```python
from build123d import *

# Parameters (mm, degrees)
F0_W        = 119.0486699343
F0_H        = 122.4547103047
F1_DEPTH    = 25.4
F2_T1_DEPTH = 131.7486699343
F2_T3_DEPTH = 135.1547103047
F3_T        = -5.08


# Not quite as in the source:
# - a fillet or chamfer that OpenCascade refuses, or shapes differently, is made with other operations: its cross-section is extruded or revolved along the edge and cut away or added


with BuildPart() as f1:
    # F0 (on Front) → F1 (new body)
    with BuildSketch(Plane.XZ):
        Rectangle(F0_W, F0_H)
    extrude(amount=F1_DEPTH)

    # F2: fillet of radius 2.54 on 4 edges, made by hand

    # F2_s2 → F2_t1 (cut)
    with BuildSketch(Plane.YZ.offset(-65.8743349671)):
        with BuildLine():
            add(Edge.make_bspline(
                [(-22.86, 61.2273551524), (-25.4, 61.2273551524), (-25.4, 58.6873551524)],
                knots=[0, 0, 0, 1, 1, 1], degree=2, weights=[1, 1, 1]))
            Line((-25.4, 58.6873551524), (-25.4, 61.2273551524))
            Line((-25.4, 61.2273551524), (-22.86, 61.2273551524))
        make_face()
        with BuildLine():
            add(Edge.make_bspline(
                [(-22.86, -61.2273551524), (-25.4, -61.2273551524), (-25.4, -58.6873551524)],
                knots=[0, 0, 0, 1, 1, 1], degree=2, weights=[1, 1, 1]))
            Line((-25.4, -58.6873551524), (-25.4, -61.2273551524))
            Line((-25.4, -61.2273551524), (-22.86, -61.2273551524))
        make_face()
    extrude(amount=F2_T1_DEPTH, mode=Mode.SUBTRACT)

    # F2_s4 → F2_t3 (cut)
    with BuildSketch(Plane.XY.offset(-67.5773551524)):
        with BuildLine():
            add(Edge.make_bspline(
                [(-59.5243349671, -22.86), (-59.5243349671, -25.4), (-56.9843349671, -25.4)],
                knots=[0, 0, 0, 1, 1, 1], degree=2, weights=[1, 1, 1]))
            Line((-56.9843349671, -25.4), (-59.5243349671, -25.4))
            Line((-59.5243349671, -25.4), (-59.5243349671, -22.86))
        make_face()
        with BuildLine():
            add(Edge.make_bspline(
                [(59.5243349671, -22.86), (59.5243349671, -25.4), (56.9843349671, -25.4)],
                knots=[0, 0, 0, 1, 1, 1], degree=2, weights=[1, 1, 1]))
            Line((56.9843349671, -25.4), (59.5243349671, -25.4))
            Line((59.5243349671, -25.4), (59.5243349671, -22.86))
        make_face()
    extrude(amount=F2_T3_DEPTH, mode=Mode.SUBTRACT)

    # F3
    f3_openings = [f1.faces().sort_by_distance(p)[0] for p in [
        (0, 0, 0),
    ]]
    offset(amount=F3_T, openings=f3_openings)


solid = f1.part
```
Source: CAD feature listing. Evaluate the final solid. Frame: model axes, mm. A direction names the side the tool comes from. Coordinates: 2 decimals unless noted, no trailing zeros. Loops run counter-clockwise (first coordinate to the right, second up) from the corner with the lowest first, then second, coordinate; pieces in that order, holes last. Notation, with made-up numbers: M 88.5,-19.75 L 135.5,-19.75 A24 cw 135.5,-4.75 Z; hole C -36.5,68.25 d7. An arc over 180 degrees is marked long. Use a Markdown table: item, result. Add a question column.
Q1. Draft query along Z for faces 1 (the flat face through (-1, -11, 61.227)), 2 (the flat face through (-1, -10, 56.147)), 3 (the flat face through (-59.524, -11, -1)). Return one class per face: pulls with the +Z half, pulls with the -Z half, needs draft (parallel to the pull), parting line crosses it, or undercut.
Q2. Section query A-A, the plane y = -4.5. Return loops of the section in (x, z), and give its area (3 significant figures).
Q3. Material intervals for L1, parallel to Z at x = 38.5, y = -17.5; L2, parallel to X at y = -14.5, z = 8.5; L3, parallel to Y at x = -6.5, z = 15, sorted ascending.
Q4. Access query for faces 4 (the flat face through (-1, -11, -61.227)), 5 (the flat face through (-54.444, -10, -1)). Directions: +Z, -Z, +X, -X, +Y, -Y. A direction counts if a zero-diameter tool reaches every point of the face in a straight line with its end or side. Return the directions, or none.
Result:
| question | item | result |
|---|---|---|
| 1 | face 1 | pulls with the +Z half |
| 1 | face 2 | undercut |
| 1 | face 3 | needs draft |
| 2 | outline | M -59.52,-61.23 L 59.52,-61.23 L 59.52,61.23 L -59.52,61.23 Z; hole M -54.44,-56.15 L 54.44,-56.15 L 54.44,56.15 L -54.44,56.15 Z |
| 2 | area | 2,350 mm2 |
| 3 | L1 | z = -61.23 to -56.15, 56.15 to 61.23 |
| 3 | L2 | x = -59.52 to -54.44, 54.44 to 59.52 |
| 3 | L3 | y = -25.4 to -20.32 |
| 4 | face 4 | -Z, +X, -X, +Y, -Y |
| 4 | face 5 | +Y |
